Drawing for the job (mm, zero at the part's lowest x, y, z). Give positions to 0.01 mm unless a question says otherwise; leave off trailing zeros. Order: outer loops, then holes, each group sorted by start corner. A loop starts at its lowest first (then second) coordinate and runs counter-clockwise, first axis right, second up. Notation, with made-up numbers: (67, -3.5) - (100, -3.5) arc R34 ccw to (100, 28.5) - close; hole circle Ø6 at (28.5, -10.5). An arc over 180 degrees is marked (long way). Use a Markdown table: item, result. Add a question column.
(1) Slice it at A-A (x = 9). Write the cut outline in (y, z), then the cut area to 3 significant figures.
(2) Slice it at C-C (y = 4). Count the separate pieces of the cut face and the enclosed holes in it, then the cut area to 3 significant figures.
(3) Flat gauge pin, fed straight in: pin 1 (2.5 mm diameter, centred on x = 29, z = 4, fed in from +Y). Where does the tip first touch, or does it go through?
(4) Wall check: line 1 (X direction, y = 3.5, z = 4); line 2 (X direction, y = 0.5, z = 2.25); line 3 (Z direction, x = 29, y = 4.5). Give the ranges that are in metal, low to high.
(5) Slice it at B-B (z = 2.75). Write the cut outline in (x, y).
(6) Mould opens along X. For the marked faces 1, 2 and 3 say: +X half, -X half, draft (parallel to the pull), parting line (faces both ways), or undercut.
(7) Slice it at D-D (z = 5). Write the cut outline in (x, y).
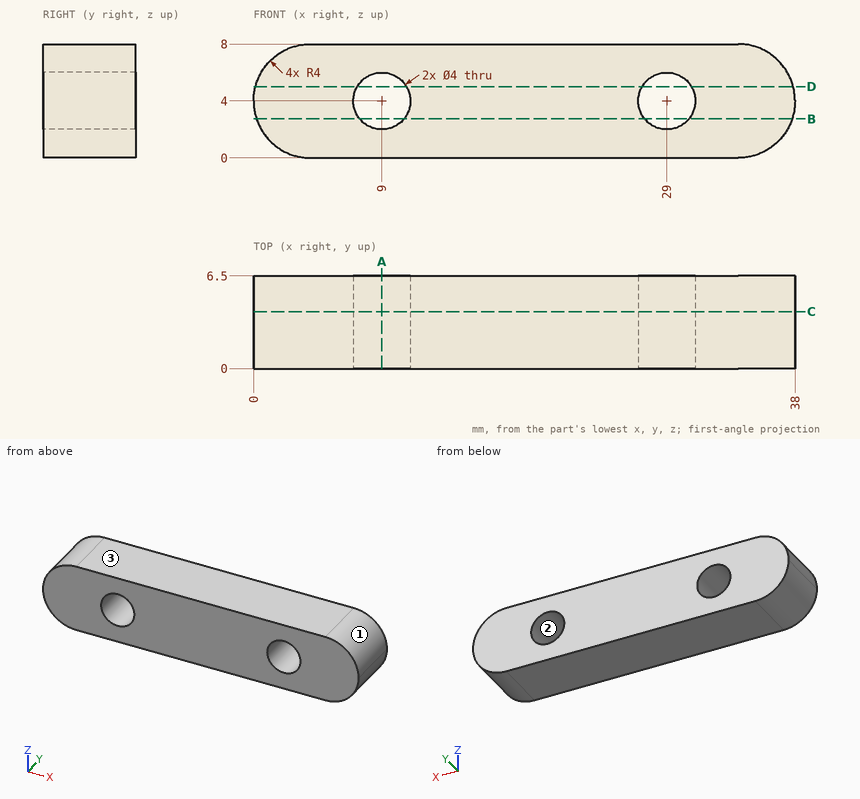
Solution:
| question | item | result |
|---|---|---|
| 1 | outline | (0, 0) - (6.5, 0) - (6.5, 2) - (0, 2) - close; (0, 6) - (6.5, 6) - (6.5, 8) - (0, 8) - close |
| 1 | area | 26.0 mm2 |
| 2 | separate pieces | 1 |
| 2 | enclosed holes | 2 |
| 2 | area | 265 mm2 |
| 3 | pin 1 | through |
| 4 | line 1 | 0 to 7, 11 to 27, 31 to 38 |
| 4 | line 2 | 0.4 to 8.03, 9.97 to 28.03, 29.97 to 37.6 |
| 4 | line 3 | 0 to 2, 6 to 8 |
| 5 | outline | (0.2, 0) - (7.44, 0) - (7.44, 6.5) - (0.2, 6.5) - close; (10.56, 0) - (27.44, 0) - (27.44, 6.5) - (10.56, 6.5) - close; (30.56, 0) - (37.8, 0) - (37.8, 6.5) - (30.56, 6.5) - close |
| 6 | face 1 | +X half |
| 6 | face 2 | undercut |
| 6 | face 3 | draft |
| 7 | outline | (0.13, 0) - (7.27, 0) - (7.27, 6.5) - (0.13, 6.5) - close; (10.73, 0) - (27.27, 0) - (27.27, 6.5) - (10.73, 6.5) - close; (30.73, 0) - (37.87, 0) - (37.87, 6.5) - (30.73, 6.5) - close |
